Input: dimensioned drawing with shaded views. Units: mm. Origin: part minimum x, y, z. A direction names the side the tool comes from. Coordinates: 2 decimals unless noted, no trailing zeros. Order: outer loops, then holes, each group sorted by start corner. A loop starts at its lowest first (then second) coordinate and runs counter-clockwise, first axis right, second up.
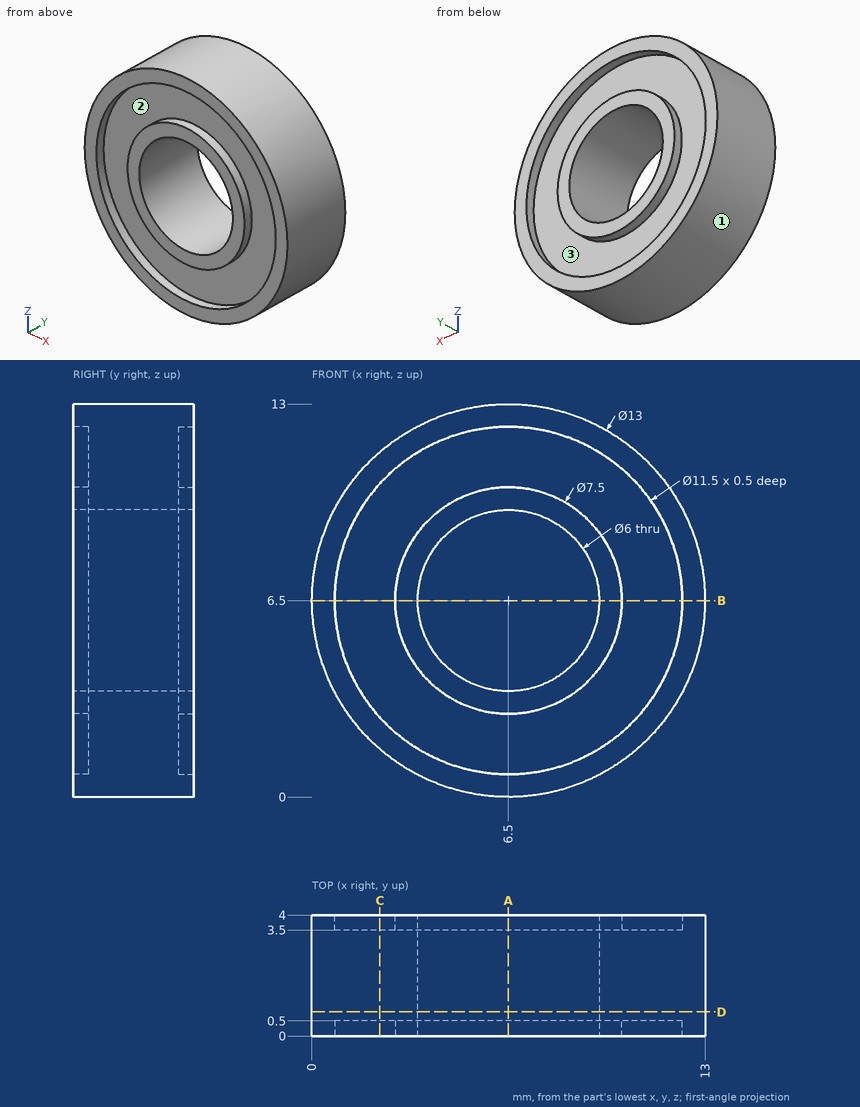
1. Section query D-D on y = 0.8. Return loops of the section in (x, z), plus the area to 3 significant figures.
Findings:
outline: circle Ø13 at (6.5, 6.5); hole circle Ø6 at (6.5, 6.5)
area: 104 mm2
2. Ray query, line 1 (Z direction, x = 6.5, y = 3.85); line 2 (Z direction, x = 6.5, y = 1.75); line 3 (X direction, y = 3.7, z = 7.25). Return the intervals inside material, ascending.
Findings:
line 1: z = 0 to 0.75, 2.75 to 3.5, 9.5 to 10.25, 12.25 to 13
line 2: z = 0 to 3.5, 9.5 to 13
line 3: x = 0.04 to 0.8, 2.83 to 3.6, 9.4 to 10.17, 12.2 to 12.96
3. Section query B-B on z = 6.5. Return loops of the section in (x, y).
Findings:
outline: (0, 0) - (0.75, 0) - (0.75, 0.5) - (2.75, 0.5) - (2.75, 0) - (3.5, 0) - (3.5, 4) - (2.75, 4) - (2.75, 3.5) - (0.75, 3.5) - (0.75, 4) - (0, 4) - close; (9.5, 0) - (10.25, 0) - (10.25, 0.5) - (12.25, 0.5) - (12.25, 0) - (13, 0) - (13, 4) - (12.25, 4) - (12.25, 3.5) - (10.25, 3.5) - (10.25, 4) - (9.5, 4) - close
4. Access query for the marked faces 1, 2 and 3. Directions: +Z, -Z, +X, -X, +Y, -Y. A direction counts if a zero-diameter tool reaches every point of the face in a straight line with its end or side. Return the directions, or none.
Findings:
face 1: +Y, -Y
face 2: -Y
face 3: +Y
5. Section query C-C on x = 2.25. Return loops of the section in (y, z).
Findings:
outline: (0, 1.58) - (4, 1.58) - (4, 2.63) - (3.5, 2.63) - (3.5, 10.37) - (4, 10.37) - (4, 11.42) - (0, 11.42) - (0, 10.37) - (0.5, 10.37) - (0.5, 2.63) - (0, 2.63) - close
6. Pin query (flat end, axial travel): P1, Ø2, axis at y = 0.5, z = 4, coming from the -X side; P2, Ø1, axis at x = 3, y = 1, coming from the -Z side. Return the tip coordinate at first contact, or that it passes through.
Findings:
P1: stops at x = 0.18
P2: stops at z = 0.73
7. Section query A-A on x = 6.5. Return loops of the section in (y, z), plus the area to 3 significant figures.
Findings:
outline: (0, 0) - (4, 0) - (4, 0.75) - (3.5, 0.75) - (3.5, 2.75) - (4, 2.75) - (4, 3.5) - (0, 3.5) - (0, 2.75) - (0.5, 2.75) - (0.5, 0.75) - (0, 0.75) - close; (0, 9.5) - (4, 9.5) - (4, 10.25) - (3.5, 10.25) - (3.5, 12.25) - (4, 12.25) - (4, 13) - (0, 13) - (0, 12.25) - (0.5, 12.25) - (0.5, 10.25) - (0, 10.25) - close
area: 24.0 mm2
